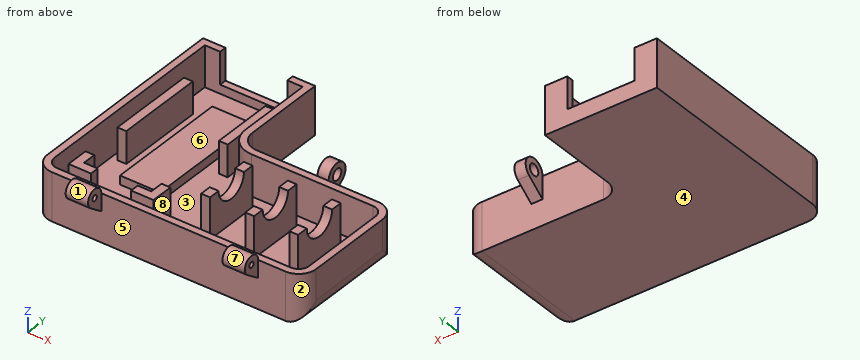
```python
from build123d import *

# Parameters (mm, degrees)
SALIENTE_EXTRUIR1_DEPTH = 54.1
REDONDEO1_R             = 10
CROQUIS2_W              = 27.05
CROQUIS2_H              = 127
CORTAR_EXTRUIR1_DEPTH   = 206.624828267
VACIADO1_T              = -4
CROQUIS3_W              = 22.730580246
CROQUIS3_H              = 69.392963169
SALIENTE_EXTRUIR2_DEPTH = 5
CROQUIS3_3_W            = 5
CROQUIS3_3_H            = 50
CROQUIS3_3_H_2          = 35
SALIENTE_EXTRUIR3_DEPTH = 18
CROQUIS4_W              = 5
CROQUIS4_H              = 32.000123075
SALIENTE_EXTRUIR4_DEPTH = 23.05
CORTAR_EXTRUIR2_REACH   = 185.317
CROQUIS5_R              = 9.525
CROQUIS6_W              = 38.1
CROQUIS6_H              = 42.277753805
CORTAR_EXTRUIR3_DEPTH   = 18
SALIENTE_EXTRUIR5_DEPTH = 12.7
SALIENTE_EXTRUIR6_START = -12.7
SALIENTE_EXTRUIR6_DEPTH = 12.7
CROQUIS9_R              = 1.5875
CORTAR_EXTRUIR4_DEPTH   = 183.442326503
CROQUIS10_R             = 3.175
SALIENTE_EXTRUIR7_DEPTH = 6.35


with BuildPart() as part:
    # Croquis1 → Saliente-Extruir1 (new body)
    with BuildSketch(Plane.XY):
        Polygon((0, 0), (0, 127), (63.5, 127), (63.5, 69.85), (152.4, 69.85), (152.4, 0), align=None)
    extrude(amount=SALIENTE_EXTRUIR1_DEPTH)

    # Redondeo1
    redondeo1_edges = [part.edges().sort_by_distance(p)[0] for p in [
        (63.5, 69.85, 27.05),
        (152.4, 69.85, 27.05),
        (152.4, 0, 27.05),
        (0, 0, 27.05),
        (152.4, 34.925, 0),
    ]]
    fillet(redondeo1_edges, radius=REDONDEO1_R)

    # Croquis2 → Cortar-Extruir1 (cut, through all)
    with BuildSketch(Plane(origin=(152.4, 0, 0), x_dir=(0, 0, -1), z_dir=(1, 0, 0))):
        with Locations((-40.575, 63.5)):
            Rectangle(CROQUIS2_W, CROQUIS2_H)
    extrude(amount=-CORTAR_EXTRUIR1_DEPTH, mode=Mode.SUBTRACT)

    # Vaciado1
    vaciado1_openings = [part.faces().sort_by_distance(p)[0] for p in [
        (64.737748774, 51.223088278, 27.05),
    ]]
    offset(amount=VACIADO1_T, openings=vaciado1_openings)

    # Croquis3 → Saliente-Extruir2 (add)
    with BuildSketch(Plane.XY.offset(4)):
        with Locations((31.75, 72.216754897)):
            Rectangle(CROQUIS3_W, CROQUIS3_H)
    extrude(amount=SALIENTE_EXTRUIR2_DEPTH)

    # Croquis3<3> → Saliente-Extruir3 (add)
    with BuildSketch(Plane.XY.offset(4)):
        with Locations((10.184709877, 77.438130808)):
            Rectangle(CROQUIS3_3_W, CROQUIS3_3_H)
        with Locations((53.315290123, 88.988130808)):
            Rectangle(CROQUIS3_3_W, CROQUIS3_3_H_2)
        Polygon((50.815290123, 20.688130808), (43.115290123, 20.688130808), (43.115290123, 15.688130808), (55.815290123, 15.688130808), (55.815290123, 28.388130808), (50.815290123, 28.388130808), align=None)
        Polygon((20.384709877, 20.688130808), (12.684709877, 20.688130808), (12.684709877, 28.388130808), (7.684709877, 28.388130808), (7.684709877, 15.688130808), (20.384709877, 15.688130808), align=None)
    extrude(amount=SALIENTE_EXTRUIR3_DEPTH)

    # Croquis4 → Saliente-Extruir4 (add)
    with BuildSketch(Plane.XY.offset(4)):
        with Locations((76.9, 42.913130808)):
            Rectangle(CROQUIS4_W, CROQUIS4_H)
        with Locations((101.9, 42.913130808)):
            Rectangle(CROQUIS4_W, CROQUIS4_H)
        with Locations((126.9, 42.913130808)):
            Rectangle(CROQUIS4_W, CROQUIS4_H)
    extrude(amount=SALIENTE_EXTRUIR4_DEPTH)

    # Cortar-Extruir2: up to this face of the body (flat: up to its plane)
    cortar_extruir2_end = Plane(part.part.faces().sort_by_distance((55.815290123, 22.038130808, 13))[0])
    # Croquis5 → Cortar-Extruir2 (cut, up to the picked face)
    with BuildSketch(Plane(origin=(129.4, 0, 0), x_dir=(0, 0, -1), z_dir=(1, 0, 0)), mode=Mode.PRIVATE) as cortar_extruir2_sk1:
        with Locations((-27.05, 42.913130808)):
            Circle(CROQUIS5_R)
    cortar_extruir2_tool1 = split(extrude(cortar_extruir2_sk1.sketch, amount=-CORTAR_EXTRUIR2_REACH, mode=Mode.PRIVATE), bisect_by=cortar_extruir2_end, keep=Keep.BOTH, mode=Mode.PRIVATE)
    add(cortar_extruir2_tool1.solids().sort_by(Axis((129.4, 42.913131, 27.05), (-1, 0, 0)))[0], mode=Mode.SUBTRACT)

    # Croquis6 → Cortar-Extruir3 (cut)
    with BuildSketch(Plane.XZ.offset(-123)):
        with Locations((31.75, 30.138876903)):
            Rectangle(CROQUIS6_W, CROQUIS6_H)
    extrude(amount=-CORTAR_EXTRUIR3_DEPTH, mode=Mode.SUBTRACT)

    # Croquis7 → Saliente-Extruir5 (add)
    with BuildSketch(Plane(origin=(127, 0, 0), x_dir=(0, 0, -1), z_dir=(1, 0, 0))):
        with BuildLine():
            Line((-27.05, 0), (-17.144, 0))
            Line((-17.144, 0), (-23.027384209, -7.969606405))
            ThreePointArc((-23.027384209, -7.969606405), (-31.513632603, -7.252994449), (-27.05, 0))
        make_face()
    extrude(amount=-SALIENTE_EXTRUIR5_DEPTH)

    # Croquis8 → Saliente-Extruir6 (add)
    with BuildSketch(Plane.ZY.offset(-25.4).offset(SALIENTE_EXTRUIR6_START)):
        with BuildLine():
            Line((23.027384209, -7.969606405), (17.144, 0))
            Line((17.144, 0), (27.05, 0))
            ThreePointArc((27.05, 0), (31.513632603, -7.252994449), (23.027384209, -7.969606405))
        make_face()
    extrude(amount=SALIENTE_EXTRUIR6_DEPTH)

    # Croquis9 → Cortar-Extruir4 (cut, through all)
    with BuildSketch(Plane(origin=(127, 0, 0), x_dir=(0, 0, -1), z_dir=(1, 0, 0))):
        with Locations(Location((-27.05, -5, 0), (0, 0, 180))):
            Circle(CROQUIS9_R)
    extrude(amount=-CORTAR_EXTRUIR4_DEPTH, mode=Mode.SUBTRACT)

    # Croquis10 → Saliente-Extruir7 (add)
    with BuildSketch(Plane(origin=(107.95, 0, 0), x_dir=(0, 0, -1), z_dir=(1, 0, 0))):
        with BuildLine():
            Line((-21.97, 80.01), (-14.35, 69.85))
            Line((-14.35, 69.85), (-27.05, 69.85))
            ThreePointArc((-27.05, 69.85), (-32.729612663, 79.039806331), (-21.97, 80.01))
        make_face()
        with Locations((-27.05, 76.2)):
            Circle(CROQUIS10_R, mode=Mode.SUBTRACT)
    extrude(amount=SALIENTE_EXTRUIR7_DEPTH)


solid = part.part
```
Build history of the part. All positions in model axes, mm. Face numbers are marked on the shaded views. A direction names the side the tool comes from. Coordinates: 2 decimals unless noted, no trailing zeros. Order: outer loops, then holes, each group sorted by start corner. A loop starts at its lowest first (then second) coordinate and runs counter-clockwise, first axis right, second up.
Item 1: Drill centre lines: L1, parallel to X at y = 17, z = 10.5; L2, parallel to Y at x = 27.5, z = 6.5; L3, parallel to Y at x = 110, z = 27. Where is each one in solid material? Low to high.
Filled in:
L1: x = 0 to 4, 7.68 to 20.38, 43.12 to 55.82, 148.4 to 152.4
L2: y = 0 to 4, 37.52 to 106.91, 123 to 127
L3: y = 0 to 4, 65.85 to 73.03, 79.37 to 82.55
Item 2: Drop flat-ended pins along their axis: pin 1 Ø4 at (x, z) = (49, 23.5) entering from -Y; pin 2 Ø3 at (x, y) = (59, 107) entering from -Z; pin 3 Ø3 at (y, z) = (-3, 25.5) entering from +X; pin 4 Ø4 at (x, y) = (9.5, 87.5) entering from +Z. Give the stop position or say it passes through.
Filled in:
pin 1: stops at y = 0
pin 2: stops at z = 0
pin 3: stops at x = 127
pin 4: stops at z = 22
Item 3: Mould opens along X. For the marked faces 1, 2 and 3 say: released by +X, released by -X, zero draft, split by the parting line, or undercut.
Filled in:
face 1: zero draft
face 2: released by +X
face 3: undercut
Item 4: Saw through at C-C on x = 22.5. List the corners of the cut face in (y, z), then the cut area to 3 significant figures.
Filled in:
outline: (0, 0) - (127, 0) - (127, 9) - (123, 9) - (123, 4) - (106.91, 4) - (106.91, 9) - (37.52, 9) - (37.52, 4) - (4, 4) - (4, 27.05) - (0, 27.05) - close
area: 967 mm2
Item 5: Tool access for the marked faces 4, 5, 6, 7 and 8: list every direction of +Z, -Z, +X, -X, +Y, -Y with a clear straight run to the whole face (end or side of a thin tool).
Filled in:
face 4: -Z, +X, -X, +Y, -Y
face 5: -Z, -Y
face 6: +Z, +Y
face 7: +X, -X
face 8: +Z
Item 6: Saw through at D-D on y = 96. List the corners of the cut face in (x, z), then the cut area to 3 significant figures.
Filled in:
outline: (0, 0) - (63.5, 0) - (63.5, 27.05) - (59.5, 27.05) - (59.5, 4) - (55.82, 4) - (55.82, 22) - (50.82, 22) - (50.82, 4) - (43.12, 4) - (43.12, 9) - (20.38, 9) - (20.38, 4) - (12.68, 4) - (12.68, 22) - (7.68, 22) - (7.68, 4) - (4, 4) - (4, 27.05) - (0, 27.05) - close
area: 732 mm2
Item 7: Saw through at B-B on y = 76.2. State how many separate pieces and enclosed holes the cut face has, then the cut area to 3 significant figures.
Filled in:
separate pieces: 3
enclosed holes: 0
area: 790 mm2
